```python
from build123d import *

# Parameters (mm, degrees)
F0_R      = 50
F1_DEPTH  = 2
F2_R      = 45
F3_DEPTH  = 10
F4_R      = 50
F4_R_2    = 45
F5_DEPTH  = 2
F6_R      = 10
F7_DEPTH  = 10
F8_R      = 10
F9_DEPTH  = 10
F10_R     = 5
F11_DEPTH = 34.001
F14_R     = 2.5
F15_DEPTH = 6.6698730813


with BuildPart() as f1:
    # F0 (on Top) → F1 (new body)
    with BuildSketch(Plane.XY):
        Circle(F0_R)
    extrude(amount=F1_DEPTH)

    # F2 (on face) → F3 (join)
    with BuildSketch(Plane.XY.offset(2)):
        Circle(F2_R)
    extrude(amount=F3_DEPTH)

    # F4 (on face) → F5 (join)
    with BuildSketch(Plane.XY.offset(12)):
        Circle(F4_R)
        Circle(F4_R_2, mode=Mode.SUBTRACT)
        Circle(F4_R_2)
    extrude(amount=F5_DEPTH)

    # F6 (on face) → F7 (join)
    with BuildSketch(Plane.XY.offset(14)):
        Circle(F6_R)
    extrude(amount=F7_DEPTH)

    # F8 (on face) → F9 (join)
    with BuildSketch(Plane(origin=(0, 0, 0), x_dir=(1, 0, 0), z_dir=(0, 0, -1))):
        Circle(F8_R)
    extrude(amount=F9_DEPTH)

    # F10 (on face) → F11 (cut, through all)
    with BuildSketch(Plane.XY.offset(24)):
        Circle(F10_R)
    extrude(amount=-F11_DEPTH, mode=Mode.SUBTRACT)

    # F14 (on face) → F15 (cut, up to face)
    with BuildSketch(Plane(origin=(0, 10, 0), x_dir=(-1, 0, 0), z_dir=(0, 1, 0))):
        with Locations((0, 18.5063882234)):
            Circle(F14_R)
        with Locations((0, -5.5)):
            Circle(F14_R)
    extrude(amount=-F15_DEPTH, mode=Mode.SUBTRACT)


solid = f1.part
```
Work out the finished part from the listing and answer in its coordinate system (mm). A direction names the side the tool comes from. Give positions to 0.01 mm unless a question says otherwise; leave off trailing zeros. Order: outer loops, then holes, each group sorted by start corner. A loop starts at its lowest first (then second) coordinate and runs counter-clockwise, first axis right, second up. Notation, with made-up numbers: (-7, 62) - (46, 62) arc R19 cw to (46, 93) - close; hole circle Ø9 at (17, -9.75). An arc over 180 degrees is marked (long way). One line per item, written item: value. Start each with the question number.
1. Section B-B, the plane x = 0 is taken. Count the separate pieces of the cut face and the enclosed holes in it, then the cut area to 3 significant figures.
2. Each of these flat-tipped pins is pushed along its axis until it touches: pin 1 Ø12 at (y, z) = (35, 17) entering from +X; pin 2 Ø6 at (x, z) = (0, -5.5) entering from -Y; pin 3 Ø10 at (y, z) = (21.5, 4.5) entering from +X; pin 4 Ø1 at (x, z) = (11.5, 18.5) entering from +Y. Where does it stop, or does it pass through?
3. For a pull along X with two mould halves and no side action, classify faces 1 (the face through (1.984, 7.205, 16.985)), 2 (the face through (-5, -2, 24)), 3 (the face through (-2.17, -9.76, 18.93)) as released by +X, released by -X, zero draft, split by the parting line, or undercut.
4. Section A-A, the plane y = 0 is taken. Write down the section's boundary in (x, z).
5. Consider line 1 (Z direction, x = 0, y = 8); line 2 (Z direction, x = 25.5, y = -15); line 3 (Y direction, x = 0, z = 7). Determine where each line is inside the solid, lowest interval first.
6. Section C-C, the plane z = 7.5 is taken. Write down the section's boundary in (x, y).
7. Which of the six approach directions +Z, -Z, +X, -X, +Y, -Y give full straight-line access (tool end or side, diameter ignored) to faces 4 (the face through (20.765, -39.923, 6.93)), 5 (the face through (-1.08, -4.88, 7.24)), 6 (the face through (-1.302, -9.915, -4.93)), 7 (the face through (2, 7, -7))?
8. Section D-D, the plane x = -31.5 is taken. Write down the section's boundary in (y, z), then the cut area to 3 significant figures.
Filled sheet:
1. separate pieces: 4
1. enclosed holes: 0
1. area: 1,310 mm²
2. pin 1: x = 40.15
2. pin 2: y = -10
2. pin 3: x = 46.96
2. pin 4: through
3. face 1: undercut
3. face 2: zero draft
3. face 3: split by the parting line
4. outline: (-50, 0) - (-10, 0) - (-10, -10) - (-5, -10) - (-5, 24) - (-10, 24) - (-10, 14) - (-50, 14) - (-50, 12) - (-45, 12) - (-45, 2) - (-50, 2) - close; (5, -10) - (10, -10) - (10, 0) - (50, 0) - (50, 2) - (45, 2) - (45, 12) - (50, 12) - (50, 14) - (10, 14) - (10, 24) - (5, 24) - close
5. line 1: -10 to -8, -3 to 16.01, 21.01 to 24
5. line 2: 0 to 14
5. line 3: -45 to -5, 5 to 45
6. outline: circle Ø90 at (0, 0); hole circle Ø10 at (0, 0)
7. face 4: none
7. face 5: +Z, -Z
7. face 6: -Z
7. face 7: +Y
8. outline: (-38.83, 0) - (38.83, 0) - (38.83, 2) - (32.14, 2) - (32.14, 12) - (38.83, 12) - (38.83, 14) - (-38.83, 14) - (-38.83, 12) - (-32.14, 12) - (-32.14, 2) - (-38.83, 2) - close
8. area: 953 mm²
